```python
from build123d import *

# Parameters (mm, degrees)
SKETCH1_14_W         = 241.554
SKETCH1_14_H         = 125.149549896
BOSS_EXTRUDE9_DEPTH  = 3.81
SKETCH1_W            = 241.554
SKETCH1_H            = 125.149549896
SKETCH1_W_2          = 228.854
SKETCH1_H_2          = 108.639549896
BOSS_EXTRUDE10_DEPTH = 9.171821007
SKETCH29_R           = 1.61811024
CUT_EXTRUDE12_DEPTH  = 1.5
LPATTERN24_COUNT     = 3
LPATTERN24_PITCH     = 50.8
LPATTERN25_COUNT     = 3
LPATTERN25_PITCH     = 50.8
SKETCH30_R           = 1.5
CUT_EXTRUDE13_DEPTH  = 1
LPATTERN26_COUNT     = 3
LPATTERN26_PITCH     = 50.8
LPATTERN27_COUNT     = 3
LPATTERN27_PITCH     = 50.8
SKETCH37_W           = 228.854
SKETCH37_H           = 108.639549896
BOSS_EXTRUDE12_DEPTH = 18.034
FILLET7_R            = 5.08
SKETCH38_W           = 218.694
SKETCH38_H           = 98.479549896
CUT_EXTRUDE14_DEPTH  = 8.862178993
CUT_EXTRUDE15_DEPTH  = 5.08
SURFACECUT1_START    = -3.81
SURFACECUT1_DEPTH    = 21.844


# Read off the part's stored shape, not the designer's step: SurfaceCut1
with BuildPart() as part:
    # Sketch1<14> → Boss-Extrude9 (new body)
    with BuildSketch(Plane(origin=(0, 0, 0), x_dir=(1, 0, 0), z_dir=(0, 1, 0))):
        with Locations((0, -1.905)):
            Rectangle(SKETCH1_14_W, SKETCH1_14_H)
    extrude(amount=-BOSS_EXTRUDE9_DEPTH)

    # Sketch1 → Boss-Extrude10 (add)
    with BuildSketch(Plane(origin=(0, 0, 0), x_dir=(1, 0, 0), z_dir=(0, 1, 0))):
        with Locations((0, -1.905)):
            Rectangle(SKETCH1_W, SKETCH1_H)
        Rectangle(SKETCH1_W_2, SKETCH1_H_2, mode=Mode.SUBTRACT)
    extrude(amount=BOSS_EXTRUDE10_DEPTH)

    # Sketch29 → Cut-Extrude12 (cut)
    with BuildSketch(Plane(origin=(0, 9.171821007, 0), x_dir=(1, 0, 0), z_dir=(0, 1, 0))):
        with Locations(Location((0, 57.494774948, 0), (0, 0, 270))):
            Circle(SKETCH29_R)
    cut_extrude12 = extrude(amount=-CUT_EXTRUDE12_DEPTH, mode=Mode.SUBTRACT)

    # LPattern24: Cut-Extrude12 ×3
    with Locations(*[(-i * LPATTERN24_PITCH, 0, 0) for i in range(1, LPATTERN24_COUNT)]):
        add(cut_extrude12, mode=Mode.SUBTRACT)

    # LPattern25: Cut-Extrude12 ×3
    with Locations(*[(i * LPATTERN25_PITCH, 0, 0) for i in range(1, LPATTERN25_COUNT)]):
        add(cut_extrude12, mode=Mode.SUBTRACT)

    # Sketch30 → Cut-Extrude13 (cut)
    with BuildSketch(Plane(origin=(0, 9.171821007, 0), x_dir=(1, 0, 0), z_dir=(0, 1, 0))):
        with Locations(Location((0, -59.399774948, 0), (0, 0, 270))):
            Circle(SKETCH30_R)
    cut_extrude13 = extrude(amount=-CUT_EXTRUDE13_DEPTH, mode=Mode.SUBTRACT)

    # LPattern26: Cut-Extrude13 ×3
    with Locations(*[(i * LPATTERN26_PITCH, 0, 0) for i in range(1, LPATTERN26_COUNT)]):
        add(cut_extrude13, mode=Mode.SUBTRACT)

    # LPattern27: Cut-Extrude13 ×3
    with Locations(*[(-i * LPATTERN27_PITCH, 0, 0) for i in range(1, LPATTERN27_COUNT)]):
        add(cut_extrude13, mode=Mode.SUBTRACT)

    # Sketch37 → Boss-Extrude12 (add)
    with BuildSketch(Plane(origin=(0, 0, 0), x_dir=(1, 0, 0), z_dir=(0, 1, 0))):
        Rectangle(SKETCH37_W, SKETCH37_H)
    extrude(amount=BOSS_EXTRUDE12_DEPTH)

    # Fillet7
    fillet7_edges = [part.edges().sort_by_distance(p)[0] for p in [
        (120.777, -3.81, 1.905),
        (0, -3.81, -60.669774948),
        (-120.777, -3.81, 1.905),
        (0, -3.81, 64.479774948),
        (-120.777, 2.680910504, -60.669774948),
        (-114.427, 13.602910504, -54.319774948),
        (120.777, 2.680910504, -60.669774948),
        (-114.427, 13.602910504, 54.319774948),
        (114.427, 13.602910504, 54.319774948),
        (114.427, 13.602910504, -54.319774948),
        (-114.427, 18.034, 0),
        (0, 18.034, 54.319774948),
        (114.427, 18.034, 0),
        (120.777, 2.680910504, 64.479774948),
        (0, 18.034, -54.319774948),
        (-120.777, 2.680910504, 64.479774948),
    ]]
    fillet(fillet7_edges, radius=FILLET7_R)

    # Sketch38 → Cut-Extrude14 (cut)
    with BuildSketch(Plane(origin=(0, 18.034, 0), x_dir=(1, 0, 0), z_dir=(0, 1, 0))):
        Rectangle(SKETCH38_W, SKETCH38_H)
    extrude(amount=-CUT_EXTRUDE14_DEPTH, mode=Mode.SUBTRACT)

    # Sketch40 → Cut-Extrude15 (cut)
    with BuildSketch(Plane.XZ.offset(3.81)):
        Polygon((-35.878101968, 30.590802731), (120.777, 30.590802731), (120.777, 20.320819759), (-25.608118996, 20.320819759), (-25.608118996, 13.474164444), (-4.307413572, 13.474164444), (-4.307413572, 3.204181472), (-25.608118996, 3.204181472), (-25.608118996, -3.642473843), (-4.307413572, -3.642473843), (-4.307413572, -13.912456815), (-35.878101968, -13.912456815), align=None)
        Polygon((35.878101968, -3.204181472), (12.295330254, -3.204181472), (12.295330254, 3.642473843), (35.878101968, 3.642473843), (35.878101968, 13.912456815), (2.025195134, 13.912456815), (2.025195134, -13.474164444), (25.608118996, -13.474164444), (25.608118996, -20.320667611), (-120.777, -20.320667611), (-120.777, -30.590802731), (35.878101968, -30.590802731), align=None)
    extrude(amount=-CUT_EXTRUDE15_DEPTH, mode=Mode.SUBTRACT)

    # SurfaceCut1 outline → SurfaceCut1 (cut)
    with BuildSketch(Plane(origin=(0, 0, 0), x_dir=(1, 0, 0), z_dir=(0, 1, 0)).offset(SURFACECUT1_START)):
        with BuildLine():
            Line((0, -64.479774948), (115.697, -64.479774948))
            ThreePointArc((115.697, -64.479774948), (119.289102448, -62.991877396), (120.777, -59.399774948))
            Line((120.777, -59.399774948), (120.777, 55.589774948))
            ThreePointArc((120.777, 55.589774948), (119.289102448, 59.181877396), (115.697, 60.669774948))
            Line((115.697, 60.669774948), (0, 60.669774948))
            add(Edge.make_bspline(
                [(0, 60.669774948), (-4.900958952, 48.738988323), (-8.678459932, 38.81495371), (-11.504191584, 30.590802731)],
                knots=[0.996302642, 0.996302642, 0.996302642, 0.996302642, 1.072713483, 1.072713483, 1.072713483, 1.072713483], degree=3))
            add(Edge.make_bspline(
                [(-11.504191584, 30.590802731), (-18.142241768, 11.271088885), (-19.527974886, 1.332143628), (-17.887110358, -3.204181472)],
                knots=[0.888553663, 0.888553663, 0.888553663, 0.888553663, 1.068053721, 1.068053721, 1.068053721, 1.068053721], degree=3))
            add(Edge.make_bspline(
                [(-17.887110358, -3.204181472), (-11.085165947, -22.008799781), (47.725405996, 52.02444551), (0, -64.479774948)],
                knots=[0.478911773, 0.478911773, 0.478911773, 0.478911773, 1.223000875, 1.223000875, 1.223000875, 1.223000875], degree=3))
        make_face()
    extrude(amount=SURFACECUT1_DEPTH, mode=Mode.SUBTRACT)


solid = part.part
```
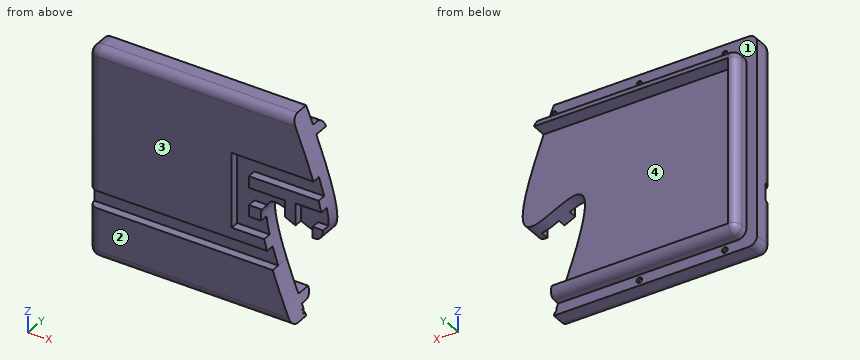
The model under review builds one solid part; all positions refer to its coordinate system, in mm. Face numbers are marked on the shaded views. A direction names the side the tool comes from. Give positions to 0.01 mm unless a question says otherwise; leave off trailing zeros. Loops run counter-clockwise (first coordinate to the right, second up) from the corner with the lowest first, then second, coordinate; pieces in that order, holes last. Notation, with made-up numbers: (64, 74) - (102, 74) arc R19 cw to (102, 96) - close; hole circle Ø7 at (32, 46.25). An arc over 180 degrees is marked (long way). Answer as a JSON object with one key per item and string values.
Q1. Mouldability with a two-part tool opening along Z and no side actions: class the marked faces 3 and 4 as +Z half, -Z half, draft (parallel to the pull), parting line (faces both ways), or undercut.
Worked out:
{"face 3": "draft", "face 4": "undercut"}
Q2. Insertion check: pin 1 (1.5 mm diameter, centred on x = -0.5, z = 59.5, fed in from +Y); pin 2 (3 mm diameter, centred on y = 13.5, z = 45, fed in from -X); pin 3 (2.5 mm diameter, centred on x = -53.5, y = -1, fed in from +Z). Each pin has a flat end and moves straight along its axis. Give the tip position at first contact, or say it passes through.
Worked out:
{"pin 1": "stops at y = 8.17", "pin 2": "stops at x = -114.43", "pin 3": "stops at z = 64.38"}
Q3. For the marked faces 1 and 2, list the 3-axis set-ups (+Z, -Z, +X, -X, +Y, -Y) from which the entire face can be reached by the end or side of a thin tool; tool diameter is ignored.
Worked out:
{"face 1": "-X, +Y", "face 2": "+Z, -Z, +X, -X, -Y"}
Q4. To check wall thickness, follow line 1 along Z through (x, y) = (-101.6, 8.65); line 2 along Z through (x, y) = (-43.5, 13.5); line 3 along Y through (x, z) = (-53, -46.5). State the ranges of each line that lie inside material, in increasing order.
Worked out:
{"line 1": "z = -60.67 to -59.11, -55.88 to 57.9, 60.9 to 64.48", "line 2": "z = -54.29 to -49.24, 49.24 to 54.29", "line 3": "y = -3.81 to 9.17"}
Q5. Add section A-A on x = -43.5. State the section outline as (y, z) points.
Worked out:
{"outline": "(-3.81, -55.59) arc R5.08 ccw to (1.27, -60.67) - (9.17, -60.67) - (9.17, -54.32) - (12.95, -54.32) arc R5.08 ccw to (18.03, -49.24) - (9.17, -49.24) - (9.17, 49.24) - (18.03, 49.24) arc R5.08 ccw to (12.95, 54.32) - (9.17, 54.32) - (9.17, 64.48) - (1.27, 64.48) arc R5.08 ccw to (-3.81, 59.4) - (-3.81, -20.32) - (1.27, -20.32) - (1.27, -30.59) - (-3.81, -30.59) - close"}
